Here's the drawing with two shaded views (mm, measured from the low corner). I have some questions. A direction names the side the tool comes from. Give positions to 0.01 mm unless a question says otherwise; leave off trailing zeros. Loops run counter-clockwise (first coordinate to the right, second up) from the corner with the lowest first, then second, coordinate; pieces in that order, holes last. Notation, with made-up numbers: M 15.5,11.5 L 35.5,11.5 A36 cw 35.5,47.5 Z; hole C -20,83 d6. An arc over 180 degrees is marked long. Use CSV: the item, a comma, the result in double quotes.
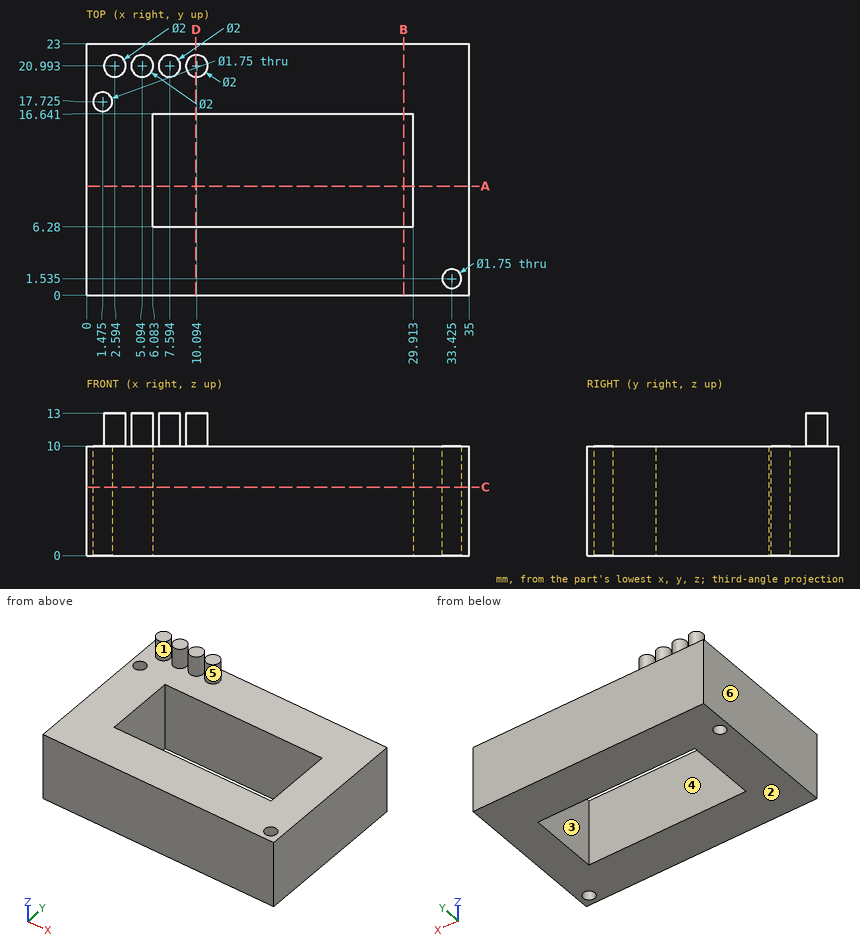
1. I want a section at C-C, the plane z = 6.25. Give the number of separate pieces and of enclosed holes in the cut face, then the cut area to 3 significant figures.
Outcome:
separate pieces,"1"
enclosed holes,"3"
area,"553 mm2"
2. I want a section at A-A, the plane y = 10. List the corners of the cut face in (x, z) for me, then the cut area to 3 significant figures.
Outcome:
outline,"M 0,0 L 6.08,0 L 6.08,10 L 0,10 Z; M 29.91,0 L 35,0 L 35,10 L 29.91,10 Z"
area,"112 mm2"
3. Please list where these lines run through material, in increasing order: line 1 (Y direction, x = 12, z = 7.25); line 2 (X direction, y = 7.75, z = 5.5); line 3 (Z direction, x = 19.5, y = 2.5).
Outcome:
line 1,"0 to 6.28, 16.64 to 23"
line 2,"0 to 6.08, 29.91 to 35"
line 3,"0 to 10"
4. I'm going to push a flat-ended pin straight in: pin 1 Ø10 at (x, y) = (16.5, 19) entering from +Z. Where does the tip first touch, or does it pass through?
Outcome:
pin 1,"z = 10"
5. I want a section at D-D, the plane x = 10. List the corners of the cut face in (y, z) for me.
Outcome:
outline,"M 0,0 L 6.28,0 L 6.28,10 L 0,10 Z; M 16.64,0 L 23,0 L 23,10 L 21.99,10 L 21.99,13 L 20,13 L 20,10 L 16.64,10 Z"
6. If we mould it in two halves opening along Y, with no side actions, what happens to the marked faces 1, 2 and 3? For each: +Y half, -Y half, draft (parallel to the pull), parting line (faces both ways), or undercut.
Outcome:
face 1,"parting line"
face 2,"draft"
face 3,"undercut"
7. I want a section at B-B, the plane x = 29. List the corners of the cut face in (y, z) for me.
Outcome:
outline,"M 0,0 L 6.28,0 L 6.28,10 L 0,10 Z; M 16.64,0 L 23,0 L 23,10 L 16.64,10 Z"
8. Which directions (+Z, -Z, +X, -X, +Y, -Y) give clear straight access to the entire face, cutting with the end or side of a thin tool? Please do the marked faces 4, 5 and 6.
Outcome:
face 4,"+Z, -Z"
face 5,"+Z"
face 6,"+Z, -Z, -X, +Y, -Y"
